Source: CAD feature listing. Evaluate the final solid. Frame: model axes, mm. A direction names the side the tool comes from. Give positions to 0.01 mm unless a question says otherwise; leave off trailing zeros. Loops run counter-clockwise (first coordinate to the right, second up) from the corner with the lowest first, then second, coordinate; pieces in that order, holes last. Notation, with made-up numbers: (49.5, 22) - (103.5, 22) arc R34 ccw to (103.5, 58) - close; hole circle Ø7 at (37, -23.5). An arc over 180 degrees is marked (long way). Write each question's results on one line, items separated by ' | '. Start each with the question number.
(1) Reachability of faces 1 (the flat face through (0, -2.652, -3)), 2 (the flat face through (2.652, 0, 13)), 3 (the flat face through (0, 2.652, 13)), 4 (the flat face through (0, 2.652, -3)) from +Z, -Z, +X, -X, +Y, -Y: full face, straight path, thin tool, end or side. Return the list, or none.
(2) Cut plane D-D on x = -2. Return the cut outline in (y, z), then the cut area to 3 significant figures.
(3) Contact query for flat-ended pins moving along their axis: pin 1 (1.2 mm diameter, centred on x = -0.5, z = 13.5, fed in from +Y); pin 2 (1.2 mm diameter, centred on y = 0.5, z = 13.5, fed in from -X); pin 3 (4.5 mm diameter, centred on y = 0, z = 13, fed in from +X). Output: stop coordinate, or through.
(4) Material intervals for line 1 along Y through (x, z) = (-0.5, 11); line 2 along X through (y, z) = (1, 4.75), sorted ascending. Write a range as [from, to].
(5) Cut plane C-C on z = -1.75. Return the cut outline in (x, y).
(6) Cut plane A-A on y = 0. Return the cut outline in (x, z).
from build123d import *

# Parameters (mm, degrees)
SKETCH2_R           = 3.75
BOSS_EXTRUDE1_DEPTH = 10
SKETCH3_W           = 5.303300858
SKETCH3_H           = 5.303300858
BOSS_EXTRUDE2_DEPTH = 5
SKETCH4_W           = 5.303300858
SKETCH4_H           = 5.303300858
BOSS_EXTRUDE3_DEPTH = 5
FILLET1_R           = 1
FILLET3_R           = 1
FILLET4_R           = 1
FILLET5_R           = 1
FILLET6_R           = 1
FILLET7_R           = 1
FILLET8_R           = 1
FILLET9_R           = 1


with BuildPart() as part:
    # Sketch2 → Boss-Extrude1 (new body)
    with BuildSketch(Plane.XY):
        Circle(SKETCH2_R)
    extrude(amount=BOSS_EXTRUDE1_DEPTH)

    # Sketch3 → Boss-Extrude2 (add)
    with BuildSketch(Plane.XY.offset(10)):
        Rectangle(SKETCH3_W, SKETCH3_H)
    extrude(amount=BOSS_EXTRUDE2_DEPTH)

    # Sketch4 → Boss-Extrude3 (add)
    with BuildSketch(Plane(origin=(0, 0, 0), x_dir=(-1, 0, 0), z_dir=(0, 0, -1))):
        Rectangle(SKETCH4_W, SKETCH4_H)
    extrude(amount=BOSS_EXTRUDE3_DEPTH)

    # Fillet1
    # the kernel refuses this fillet: 1 mm, written as the material it adds along each edge
    with BuildSketch(Plane(origin=(-2.651650429, 2.651650429, 10), x_dir=(-1, 0, 0), z_dir=(0, -1, 0))) as fillet1_piece_1_section:
        with BuildLine():
            CenterArc((FILLET1_R, -FILLET1_R), FILLET1_R, 90, 90)
            Line((0, -FILLET1_R), (0, 0))
            Line((0, 0), (FILLET1_R, 0))
        make_face()
    fillet1_piece_1 = extrude(amount=5.303300859, mode=Mode.PRIVATE)
    fillet1_piece_1 = fillet1_piece_1 & Plane(origin=(0, 0, 10.241590104), x_dir=(1, 0, 0), z_dir=(0, 0, -1)) * Cylinder(3.75, 15, mode=Mode.PRIVATE)
    add(fillet1_piece_1)

    # Fillet3
    # the kernel refuses this fillet: 1 mm, written as the material it adds along each edge
    with BuildSketch(Plane(origin=(2.651650429, 2.651650429, 10), x_dir=(0, 0, 1), z_dir=(-1, 0, 0))) as fillet3_piece_1_section:
        with BuildLine():
            CenterArc((FILLET3_R, FILLET3_R), FILLET3_R, 180, 90)
            Line((0, FILLET3_R), (0, 0))
            Line((0, 0), (FILLET3_R, 0))
        make_face()
    fillet3_piece_1 = extrude(amount=7.803300859, mode=Mode.PRIVATE)
    fillet3_piece_1 = fillet3_piece_1 & Plane(origin=(0, 0, 10.24158994), x_dir=(1, 0, 0), z_dir=(0, 0, -1)) * Cylinder(3.75, 20, mode=Mode.PRIVATE)
    add(fillet3_piece_1)

    # Fillet4
    # the kernel refuses this fillet: 1 mm, written as the material it adds along each edge
    with BuildSketch(Plane(origin=(2.651650429, -2.651650429, 10), x_dir=(0, 0, 1), z_dir=(0, 1, 0))) as fillet4_piece_1_section:
        with BuildLine():
            CenterArc((FILLET4_R, FILLET4_R), FILLET4_R, 180, 90)
            Line((0, FILLET4_R), (0, 0))
            Line((0, 0), (FILLET4_R, 0))
        make_face()
    fillet4_piece_1 = extrude(amount=7.803300859, mode=Mode.PRIVATE)
    fillet4_piece_1 = fillet4_piece_1 & Plane(origin=(0, 0, 10.24158994), x_dir=(1, 0, 0), z_dir=(0, 0, -1)) * Cylinder(3.75, 20, mode=Mode.PRIVATE)
    add(fillet4_piece_1)

    # Fillet5
    fillet5_edges = [part.edges().sort_by_distance(p)[0] for p in [
        (0, -2.651650429, 10),
    ]]
    fillet(fillet5_edges, radius=FILLET5_R)

    # Fillet6
    # the kernel refuses this fillet: 1 mm, written as the material it adds along each edge
    with BuildSketch(Plane(origin=(-2.651650429, 2.651650429, 0), x_dir=(0, 1, 0), z_dir=(1, 0, 0))) as fillet6_piece_1_section:
        with BuildLine():
            CenterArc((FILLET6_R, -FILLET6_R), FILLET6_R, 90, 90)
            Line((0, -FILLET6_R), (0, 0))
            Line((0, 0), (FILLET6_R, 0))
        make_face()
    fillet6_piece_1 = extrude(amount=5.303300859, mode=Mode.PRIVATE)
    fillet6_piece_1 = fillet6_piece_1 & Plane(origin=(0, 0, -0.241590055), x_dir=(1, 0, 0), z_dir=(0, 0, -1)) * Cylinder(3.75, 15, mode=Mode.PRIVATE)
    add(fillet6_piece_1)

    # Fillet7
    # the kernel refuses this fillet: 1 mm, written as the material it adds along each edge
    with BuildSketch(Plane(origin=(-2.651650429, -2.651650429, 0), x_dir=(0, 0, -1), z_dir=(0, 1, 0))) as fillet7_piece_1_section:
        with BuildLine():
            CenterArc((FILLET7_R, FILLET7_R), FILLET7_R, 180, 90)
            Line((0, FILLET7_R), (0, 0))
            Line((0, 0), (FILLET7_R, 0))
        make_face()
    fillet7_piece_1 = extrude(amount=7.803300859, mode=Mode.PRIVATE)
    fillet7_piece_1 = fillet7_piece_1 & Plane(origin=(0, 0, -0.241590003), x_dir=(1, 0, 0), z_dir=(0, 0, -1)) * Cylinder(3.75, 20, mode=Mode.PRIVATE)
    add(fillet7_piece_1)

    # Fillet8
    # the kernel refuses this fillet: 1 mm, written as the material it adds along each edge
    with BuildSketch(Plane(origin=(2.651650429, -2.651650429, 0), x_dir=(0, 0, -1), z_dir=(-1, 0, 0))) as fillet8_piece_1_section:
        with BuildLine():
            CenterArc((FILLET8_R, FILLET8_R), FILLET8_R, 180, 90)
            Line((0, FILLET8_R), (0, 0))
            Line((0, 0), (FILLET8_R, 0))
        make_face()
    fillet8_piece_1 = extrude(amount=7.803300859, mode=Mode.PRIVATE)
    fillet8_piece_1 = fillet8_piece_1 & Plane(origin=(0, 0, -0.241589985), x_dir=(1, 0, 0), z_dir=(0, 0, -1)) * Cylinder(3.75, 20, mode=Mode.PRIVATE)
    add(fillet8_piece_1)

    # Fillet9
    fillet9_edges = [part.edges().sort_by_distance(p)[0] for p in [
        (2.651650429, 0, 0),
    ]]
    fillet(fillet9_edges, radius=FILLET9_R)


solid = part.part
Ans:
1) face 1: -Z, +X, -X, -Y | face 2: +Z, +X, +Y, -Y | face 3: +Z, +X, -X, +Y | face 4: -Z, +X, -X, +Y
2) outline: (-3.17, -0.12) arc R1 cw to (-2.65, -1) - (-2.65, -5) - (2.65, -5) - (2.65, -1) arc R1 cw to (3.17, -0.12) - (3.17, 10.12) arc R1 cw to (2.65, 11) - (2.65, 15) - (-2.65, 15) - (-2.65, 11) arc R1 cw to (-3.17, 10.12) - close | area: 117 mm^2
3) pin 1: y = 2.65 | pin 2: x = -2.65 | pin 3: x = 2.68
4) line 1: [-2.65, 2.65] | line 2: [-3.61, 3.61]
5) outline: (-2.65, -2.65) - (2.65, -2.65) - (2.65, 2.65) - (-2.65, 2.65) - close
6) outline: (-3.75, 0) - (-3.65, 0) arc R1 cw to (-2.65, -1) - (-2.65, -5) - (2.65, -5) - (2.65, -1) arc R1 cw to (3.65, 0) - (3.75, 0) - (3.75, 10) - (3.65, 10) arc R1 cw to (2.65, 11) - (2.65, 15) - (-2.65, 15) - (-2.65, 11) arc R1 cw to (-3.65, 10) - (-3.75, 10) - close
